Can you work these out from the model? Positions are in its coordinate system, mm. Face numbers are marked on the shaded views. A direction names the side the tool comes from. Coordinates: 2 decimals unless noted, no trailing zeros. Order: outer loops, then holes, each group sorted by start corner. A loop starts at its lowest first (then second) coordinate and runs counter-clockwise, first axis right, second up. Notation, with made-up numbers: (28.25, 35.25) -> (35.25, 35.25) arc R28 ccw to (35.25, 57.25) -> close; hole circle Ø3 at (12.25, 56). An arc over 180 degrees is marked (long way). Answer in a Markdown table with one row per item. Add a question column.
1. If I drill on line 1 along Y through (x, z) = (-59.65, 38.3); line 2 along Z through (x, y) = (-34, 18.5); line 3 along Y through (x, z) = (91, 36.75), over which ranges is the centre line in solid material (lowest first)? Write a range as [from, to].
2. Imagine slicing it at A-A on z = 29. Write out the boundary of the cut face in (x, y).
3. We'd pull the mould along Z, two halves only. Please class the marked faces 1, 2, 3 and 4: pulls with the +Z half, pulls with the -Z half, needs draft (parallel to the pull), parting line crosses it, or undercut.
4. Imagine slicing it at C-C on y = 0. State how many separate pieces and enclosed holes the cut face has, plus the area to 3 significant figures.
5. On a 3-axis mill with a long thin cutter (end or side, diameter ignored), from which of +Z, -Z, +X, -X, +Y, -Y can I reach the whole of each face in a straight line? I mean the marked faces 5, 6 and 7. Say none if no direction works.
6. Imagine slicing it at B-B on y = -9. Write out the boundary of the cut face in (x, z).
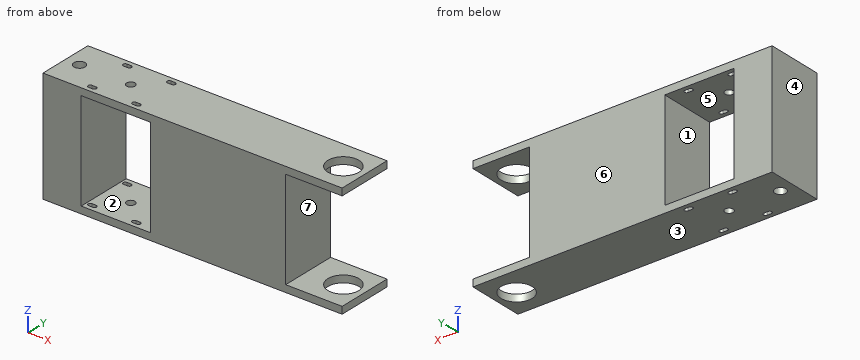
from build123d import *

# Parameters (mm, degrees)
SKETCH1_W               = 212
SKETCH1_H               = 40
SKETCH1_R               = 4
SKETCH1_R_2             = 3
SKETCH1_R_3             = 11
BOSS_EXTRUDE1_DEPTH     = 40
CUT_EXTRUDE3_DEPTH      = 116.047816146
CUT_EXTRUDE3_DEPTH_BACK = 116.047816146
SKETCH2_W               = 49
SKETCH2_H               = 70
SKETCH2_W_2             = 40


with BuildPart() as part:
    # Sketch1 → Boss-Extrude1 (new, symmetric)
    with BuildSketch(Plane.XY):
        Rectangle(SKETCH1_W, SKETCH1_H)
        with Locations((-96, 0)):
            Circle(SKETCH1_R, mode=Mode.SUBTRACT)
        with Locations((-59.65, 0)):
            Circle(SKETCH1_R_2, mode=Mode.SUBTRACT)
        with Locations((91, 0)):
            Circle(SKETCH1_R_3, mode=Mode.SUBTRACT)
        with BuildLine():
            Line((-76, 17.1), (-73, 17.1))
            ThreePointArc((-73, 17.1), (-71.5, 15.6), (-73, 14.1))
            Line((-73, 14.1), (-76, 14.1))
            ThreePointArc((-76, 14.1), (-77.5, 15.6), (-76, 17.1))
        make_face(mode=Mode.SUBTRACT)
        with BuildLine():
            Line((-44.8, 17.1), (-41.8, 17.1))
            ThreePointArc((-41.8, 17.1), (-40.3, 15.6), (-41.8, 14.1))
            Line((-41.8, 14.1), (-44.8, 14.1))
            ThreePointArc((-44.8, 14.1), (-46.3, 15.6), (-44.8, 17.1))
        make_face(mode=Mode.SUBTRACT)
        with BuildLine():
            Line((-76, -14.1), (-73, -14.1))
            ThreePointArc((-73, -14.1), (-71.5, -15.6), (-73, -17.1))
            Line((-73, -17.1), (-76, -17.1))
            ThreePointArc((-76, -17.1), (-77.5, -15.6), (-76, -14.1))
        make_face(mode=Mode.SUBTRACT)
        with BuildLine():
            Line((-44.8, -14.1), (-41.8, -14.1))
            ThreePointArc((-41.8, -14.1), (-40.3, -15.6), (-41.8, -17.1))
            Line((-41.8, -17.1), (-44.8, -17.1))
            ThreePointArc((-44.8, -17.1), (-46.3, -15.6), (-44.8, -14.1))
        make_face(mode=Mode.SUBTRACT)
    extrude(amount=BOSS_EXTRUDE1_DEPTH, both=True)

    # Sketch2 → Cut-Extrude3 (cut, two sides: drawn at the far end of the back side and taken through both)
    with BuildSketch(Plane(origin=(0, 0, 0), x_dir=(1, 0, 0), z_dir=(0, 1, 0)).offset(-CUT_EXTRUDE3_DEPTH_BACK)):
        with Locations((-54.4, 0)):
            Rectangle(SKETCH2_W, SKETCH2_H)
        with Locations((86, 0)):
            Rectangle(SKETCH2_W_2, SKETCH2_H)
    extrude(amount=CUT_EXTRUDE3_DEPTH + CUT_EXTRUDE3_DEPTH_BACK, mode=Mode.SUBTRACT)


solid = part.part
Answers follow:
| question | item | result |
|---|---|---|
| 1 | line 1 | y = [-20, -3], [3, 20] |
| 1 | line 2 | z = [-40, -35], [35, 40] |
| 1 | line 3 | y = [-20, -11], [11, 20] |
| 2 | outline | (-106, -20) -> (-78.9, -20) -> (-78.9, 20) -> (-106, 20) -> close; (-29.9, -20) -> (66, -20) -> (66, 20) -> (-29.9, 20) -> close; hole circle Ø8 at (-96, 0) |
| 3 | face 1 | undercut |
| 3 | face 2 | undercut |
| 3 | face 3 | pulls with the -Z half |
| 3 | face 4 | needs draft |
| 4 | separate pieces | 5 |
| 4 | enclosed holes | 0 |
| 4 | area | 9,810 mm² |
| 5 | face 5 | +Y, -Y |
| 5 | face 6 | +Z, -Z, +X, -X, +Y |
| 5 | face 7 | +X, +Y, -Y |
| 6 | outline | (-106, -40) -> (84.68, -40) -> (84.68, -35) -> (66, -35) -> (66, 35) -> (84.68, 35) -> (84.68, 40) -> (-106, 40) -> close; (97.32, -40) -> (106, -40) -> (106, -35) -> (97.32, -35) -> close; (97.32, 35) -> (106, 35) -> (106, 40) -> (97.32, 40) -> close; hole (-78.9, -35) -> (-29.9, -35) -> (-29.9, 35) -> (-78.9, 35) -> close |
